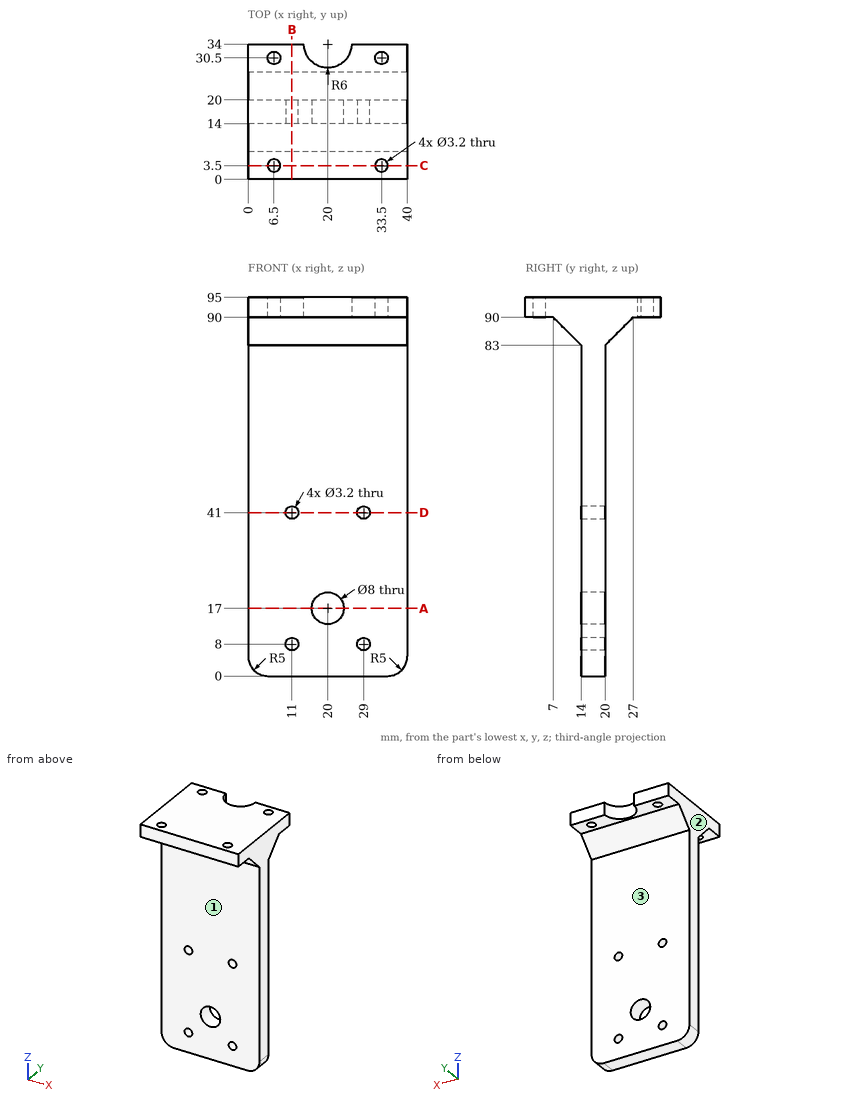
The drawing under review shows one solid part. Ordinate dimensions are in mm from its lowest x, y, z. A direction names the side the tool comes from. Coordinates: 2 decimals unless noted, no trailing zeros. Order: outer loops, then holes, each group sorted by start corner. A loop starts at its lowest first (then second) coordinate and runs counter-clockwise, first axis right, second up. Notation, with made-up numbers: (52, 73) -> (60, 73) arc R19 cw to (60, 93) -> close; hole circle Ø5 at (-39, 53). An arc over 180 degrees is marked (long way). Use CSV: the item, a comma, the result in double quotes. Start each with the question number.
Item 1: For the marked faces 1, 2 and 3, list the 3-axis set-ups (+Z, -Z, +X, -X, +Y, -Y) from which the entire face can be reached by the end or side of a thin tool; tool diameter is ignored.
Item 2: We need section C-C, the plane y = 3.5. Give the boundary of the cut face in (x, z).
Item 3: We need section A-A, the plane z = 17. Give the boundary of the cut face in (x, y).
Item 4: Insertion check: pin 1 (2 mm diameter, centred on x = 17.5, y = 4.5, fed in from -Z); pin 2 (9 mm diameter, centred on x = 20, z = 17, fed in from -Y); pin 3 (20 mm diameter, centred on x = 21.5, z = 32, fed in from +Y); pin 4 (5 mm diameter, centred on y = 12.5, z = 42.5, fed in from +X). Each pin has a flat end and moves straight along its axis. Give the tip position at first contact, or say it passes through.
Item 5: We need section B-B, the plane x = 11. Give the boundary of the cut face in (y, z), then the cut area to 3 significant figures.
Item 6: Wall thickness on probe 1 along X at (y, z) = (16.9, 8); probe 2 along Z at (x, y) = (29, 18.3); probe 3 along Y at (x, z) = (26, 28.5): over which ranges is each line inside the solid? List them lowest first.
Item 7: We need section D-D, the plane z = 41. Give the boundary of the cut face in (x, y), then the cut area to 3 significant figures.
Derived:
1,face 1,"-Z, +X, -X, -Y"
1,face 2,"+Z, -Z, -X, +Y, -Y"
1,face 3,"-Z, +X, -X, +Y"
2,outline,"(0, 90) -> (4.9, 90) -> (4.9, 95) -> (0, 95) -> close; (8.1, 90) -> (31.9, 90) -> (31.9, 95) -> (8.1, 95) -> close; (35.1, 90) -> (40, 90) -> (40, 95) -> (35.1, 95) -> close"
3,outline,"(0, 14) -> (16, 14) -> (16, 20) -> (0, 20) -> close; (24, 14) -> (40, 14) -> (40, 20) -> (24, 20) -> close"
4,pin 1,"stops at z = 90"
4,pin 2,"stops at y = 14"
4,pin 3,"stops at y = 20"
4,pin 4,"stops at x = 40"
5,outline,"(0, 90) -> (7, 90) -> (14, 83) -> (14, 42.6) -> (20, 42.6) -> (20, 83) -> (27, 90) -> (34, 90) -> (34, 95) -> (0, 95) -> close; (14, 0) -> (20, 0) -> (20, 6.4) -> (14, 6.4) -> close; (14, 9.6) -> (20, 9.6) -> (20, 39.4) -> (14, 39.4) -> close"
5,area,"721 mm^2"
6,probe 1,"x = 0 to 9.4, 12.6 to 27.4, 30.6 to 40"
6,probe 2,"z = 0 to 6.4, 9.6 to 39.4, 42.6 to 95"
6,probe 3,"y = 14 to 20"
7,outline,"(0, 14) -> (9.4, 14) -> (9.4, 20) -> (0, 20) -> close; (12.6, 14) -> (27.4, 14) -> (27.4, 20) -> (12.6, 20) -> close; (30.6, 14) -> (40, 14) -> (40, 20) -> (30.6, 20) -> close"
7,area,"202 mm^2"
